Could you check a few things on this model? Use its own coordinates, in mm. A direction names the side the tool comes from. Give positions to 0.01 mm unless a question says otherwise; leave off trailing zeros. Order: outer loops, then holes, each group sorted by start corner. A loop starts at its lowest first (then second) coordinate and runs counter-clockwise, first axis right, second up. Notation, with made-up numbers: (84, 32.5) -> (128, 32.5) arc R24 cw to (128, 48.5) -> close; hole circle Ø8 at (37, 61). An arc over 180 degrees is marked (long way). One line per item, written item: value.
```python
from build123d import *

# Parameters (mm, degrees)
BOSS_EXTRUDE2_DEPTH     = 30
SKETCH1_5_R             = 11.7
BOSS_EXTRUDE3_DEPTH     = 1.6
CUT_EXTRUDE2_REACH      = 37.795
CUT_EXTRUDE2_END_RADIUS = 12.5
CUT_EXTRUDE3_REACH      = 37.795
SKETCH4_R               = 2
CUT_EXTRUDE4_DEPTH      = 42.833001458
CUT_EXTRUDE4_DEPTH_BACK = 42.833001458
SKETCH5_R               = 2


with BuildPart() as part:
    # Sketch1 → Boss-Extrude2 (new body)
    with BuildSketch(Plane(origin=(0, 0, 0), x_dir=(1, 0, 0), z_dir=(0, 1, 0))):
        with BuildLine():
            ThreePointArc((0, -11.7), (-11.7, 0), (0, 11.7))
            Line((0, 11.7), (13.4, 11.7))
            Line((13.4, 11.7), (15, 11.7))
            Line((15, 11.7), (15, 12.5))
            Line((15, 12.5), (0, 12.5))
            ThreePointArc((0, 12.5), (-12.5, 0), (0, -12.5))
            Line((0, -12.5), (15, -12.5))
            Line((15, -12.5), (15, -11.7))
            Line((15, -11.7), (13.4, -11.7))
            Line((13.4, -11.7), (0, -11.7))
        make_face()
    extrude(amount=BOSS_EXTRUDE2_DEPTH)

    # Sketch1<5> → Boss-Extrude3 (add)
    with BuildSketch(Plane(origin=(0, 0, 0), x_dir=(1, 0, 0), z_dir=(0, 1, 0))):
        with BuildLine():
            Line((13.4, 11.7), (0, 11.7))
            ThreePointArc((0, 11.7), (8.27314934, 8.27314934), (11.7, 0))
            ThreePointArc((11.7, 0), (8.27314934, -8.27314934), (0, -11.7))
            Line((0, -11.7), (13.4, -11.7))
            Line((13.4, -11.7), (15, -11.7))
            Line((15, -11.7), (15, 11.7))
            Line((15, 11.7), (13.4, 11.7))
        make_face()
        Circle(SKETCH1_5_R)
    extrude(amount=BOSS_EXTRUDE3_DEPTH)

    # Cut-Extrude2: up to this cylinder (the profile starts inside it)
    cut_extrude2_end = Plane(origin=(0, 20.117223, 0), z_dir=(0, -1, 0)) * Cylinder(CUT_EXTRUDE2_END_RADIUS, 101.59, mode=Mode.PRIVATE)
    # Sketch3 → Cut-Extrude2 (cut, up to the surface)
    with BuildSketch(Plane(origin=(0, 0, 0), x_dir=(0, 0, -1), z_dir=(1, 0, 0)), mode=Mode.PRIVATE) as cut_extrude2_sk1:
        with BuildLine():
            Line((-11.7, 30), (11.7, 30))
            add(Edge.make_bspline(
                [(-11.7, 30), (0, -19.413885882), (11.7, 30)],
                knots=[0, 0, 0, 1, 1, 1], degree=2))
        make_face()
    cut_extrude2_tool1 = extrude(cut_extrude2_sk1.sketch, amount=-CUT_EXTRUDE2_REACH, mode=Mode.PRIVATE) & cut_extrude2_end
    add(cut_extrude2_tool1.solids().sort_by_distance((0, 20.117223, 0))[0], mode=Mode.SUBTRACT)

    # Sketch4 → Cut-Extrude3 (cut, up to next)
    with BuildSketch(Plane.XZ, mode=Mode.PRIVATE) as cut_extrude3_sk1:
        with Locations(Location((0, 0, 0), (0, 0, 270))):
            Circle(SKETCH4_R)
    cut_extrude3_tool1 = extrude(cut_extrude3_sk1.sketch, amount=-CUT_EXTRUDE3_REACH, mode=Mode.PRIVATE) & part.part
    add(cut_extrude3_tool1.solids().sort_by_distance((0, 0, 0))[0], mode=Mode.SUBTRACT)

    # Sketch5 → Cut-Extrude4 (cut, two sides: drawn at the far end of the back side and taken through both)
    with BuildSketch(Plane(origin=(0, 0, -12.5), x_dir=(-1, 0, 0), z_dir=(0, 0, -1)).offset(-CUT_EXTRUDE4_DEPTH_BACK)):
        with Locations((-6.940962405, 26.50064478)):
            Circle(SKETCH5_R)
    extrude(amount=CUT_EXTRUDE4_DEPTH + CUT_EXTRUDE4_DEPTH_BACK, mode=Mode.SUBTRACT)


solid = part.part
```
1) For P1, Ø2, axis at x = -9, y = 10.5, coming from the +Z side; P2, Ø1.5, axis at y = 4.5, z = -9, coming from the -X side; P3, Ø11.5, axis at x = 5.5, z = -3.5, coming from the +Y side; P4, Ø3.5, axis at x = 6.94, y = 26.5, coming from the +Z side, each with a flat end and sliding along its axis, tell me the tip position at first contact or that it passes through.
Answer below:
P1: stops at z = 9.6
P2: stops at x = -9.39
P3: stops at y = 1.6
P4: passes through
2) Suppose I cut it at A-A, the plane y = 2.5. Write out the boundary of the cut face in (x, z).
Answer below:
outline: (0, -12.5) -> (15, -12.5) -> (15, -11.7) -> (0, -11.7) arc R11.7 cw to (0, 11.7) -> (15, 11.7) -> (15, 12.5) -> (0, 12.5) arc R12.5 ccw to start
3) Suppose I cut it at B-B, the plane x = 10. Write out the boundary of the cut face in (y, z).
Answer below:
outline: (0, -12.5) -> (30, -12.5) -> (30, -11.7) -> (1.6, -11.7) -> (1.6, 11.7) -> (30, 11.7) -> (30, 12.5) -> (0, 12.5) -> close
4) If I drill on line 1 along Z through (x, y) = (5.75, 23); line 2 along X through (y, z) = (1.2, 0); line 3 along Y through (x, z) = (12.75, -2.5), over which ranges is the centre line in solid material (lowest first)?
Answer below:
line 1: z = -12.5 to -11.7, 11.7 to 12.5
line 2: x = -12.5 to -2, 2 to 15
line 3: y = 0 to 1.6
5) We'd pull the mould along Z, two halves only. Please class faces 1 (the cylindrical face through (-11.65, 8.12, -4.53)), 2 (the flat face through (8, 15, -12.5)), 3 (the flat face through (4, 1.6, 0)): +Z half, -Z half, draft (parallel to the pull), parting line (faces both ways), or undercut.
Answer below:
face 1: parting line
face 2: -Z half
face 3: undercut
6) For faces 4 (the cylindrical face through (-2, 1, 0)), 5 (the flat face through (7, 16, -11.7)), which set-ups out of +Z, -Z, +X, -X, +Y, -Y let a thin tool reach every point of the face, with its end or its side?
Answer below:
face 4: +Y, -Y
face 5: +X, +Y
